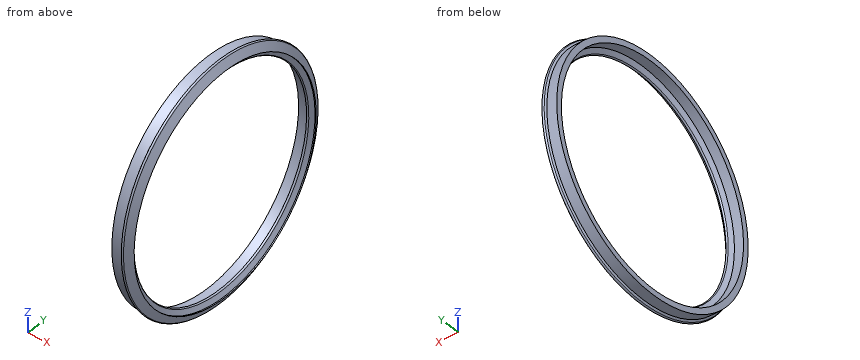
from build123d import *


with BuildPart() as part:
    # Эскиз1 → Повернуть1 (revolve)
    with BuildSketch(Plane.XY, mode=Mode.PRIVATE) as revolve_1_sk:
        with BuildLine():
            Line((0, 18.4), (1.553589838, 18.4))
            Line((1.553589838, 18.4), (1.726794919, 18.7))
            ThreePointArc((1.726794919, 18.7), (1.9, 18.8), (2.073205081, 18.7))
            Line((2.073205081, 18.7), (2.766025404, 17.5))
            Line((2.766025404, 17.5), (2.577350269, 17.5))
            Line((2.577350269, 17.5), (2.173205081, 16.8))
            ThreePointArc((2.173205081, 16.8), (2, 16.7), (1.826794919, 16.8))
            Line((1.826794919, 16.8), (1.422649731, 17.5))
            Line((1.422649731, 17.5), (0, 17.5))
            Line((0, 17.5), (0, 18.4))
        make_face()
    revolve(revolve_1_sk.sketch.rotate(Axis((0, 0, 0), (1, 0, 0)), 90), axis=Axis((0, 0, 0), (1, 0, 0)))


solid = part.part
Input: part model. Units: mm. Frame: model coordinates. Coordinates: 2 decimals unless noted, no trailing zeros. Order: outer loops, then holes, each group sorted by start corner. A loop starts at its lowest first (then second) coordinate and runs counter-clockwise, first axis right, second up. Notation, with made-up numbers: M -33,51 L -26,51 A24 ccw -26,68 Z; hole C 14.25,89 d11. An arc over 180 degrees is marked long. Write item = value, one per line. Start each with the question number.
(1) Section A-A on y = 0. Output: boundary loops of the cut face in (x, z).
(2) First-contact query: P1, Ø1.5, axis at x = 1, z = 13.5, coming from the -Y side; P2, Ø1, axis at x = 1, y = 1.5, coming from the +Z side; P3, Ø1.5, axis at x = 2.5, y = 11, coming from the -Z side. Flat tips, straight axial feed; report the tip coordinate or a pass-through.
(3) Line query: line 1 along Y through (x, z) = (0.7, 0); line 2 along Z through (x, y) = (0.2, 8); line 3 along Y through (x, z) = (0.7, -11.5). Output: solid intervals per line, ascending. Write a range as [from, to].
(4) Section C-C on x = 0.55. Output: boundary loops of the cut face in (y, z), and give its area (3 significant figures).
Result set:
q1.outline = M 0,-18.4 L 1.55,-18.4 L 1.73,-18.7 A0.2 ccw 2.07,-18.7 L 2.77,-17.5 L 2.58,-17.5 L 2.17,-16.8 A0.2 ccw 1.83,-16.8 L 1.42,-17.5 L 0,-17.5 Z; M 0,17.5 L 1.42,17.5 L 1.83,16.8 A0.2 ccw 2.17,16.8 L 2.58,17.5 L 2.77,17.5 L 2.07,18.7 A0.2 ccw 1.73,18.7 L 1.55,18.4 L 0,18.4 Z
q2.P1 = -13.27
q2.P2 = 18.37
q2.P3 = -15.6
q3.line_1 = [-18.4, -17.5], [17.5, 18.4]
q3.line_2 = [-16.57, -15.56], [15.56, 16.57]
q3.line_3 = [-14.36, -13.19], [13.19, 14.36]
q4.outline = C 0,0 d36.8; hole C 0,0 d35
q4.area = 102 mm²
